Read the model definition and answer for the solid it produces. Units are mm, in the model's axes. A direction names the side the tool comes from. Give positions to 0.01 mm unless a question says otherwise; leave off trailing zeros. Write each loop counter-clockwise with the first axis right and the second up, starting at its lowest first coordinate (ties: lowest second). Pieces come first, ordered by that corner, then holes. Notation, with made-up numbers: M -5,53.5 L 22,53.5 A18 ccw 22,75.5 Z; hole C 78.25,39 d7. An arc over 180 degrees is marked long. Answer as CSV lines item,"result". Start each with the question number.
```python
from build123d import *

# Parameters (mm, degrees)
BOSS_EXTRUDE1_DEPTH = 8
SKETCH3_W           = 84
SKETCH3_H           = 8
BOSS_EXTRUDE3_DEPTH = 3
SKETCH4_R           = 1.8
CUT_EXTRUDE1_DEPTH  = 44.9089968
SKETCH5_R           = 1.8
CUT_EXTRUDE2_DEPTH  = 44.9089968
SKETCH6_R           = 3.75
CUT_EXTRUDE3_DEPTH  = 6


with BuildPart() as part:
    # Sketch2 → Boss-Extrude1 (new body)
    with BuildSketch(Plane(origin=(0, 0, 0), x_dir=(1, 0, 0), z_dir=(0, 1, 0))):
        Polygon((-10, 0), (10, 0), (20, -10), (-20, -10), align=None)
    extrude(amount=BOSS_EXTRUDE1_DEPTH)

    # Sketch3 → Boss-Extrude3 (add)
    with BuildSketch(Plane.XY.offset(10)):
        with Locations((0, 4)):
            Rectangle(SKETCH3_W, SKETCH3_H)
    extrude(amount=-BOSS_EXTRUDE3_DEPTH)

    # Sketch4 → Cut-Extrude1 (cut, through all)
    with BuildSketch(Plane.XY.offset(10)):
        with Locations((-38.15, 4)):
            Circle(SKETCH4_R)
        with Locations((38.15, 4)):
            Circle(SKETCH4_R)
    extrude(amount=-CUT_EXTRUDE1_DEPTH, mode=Mode.SUBTRACT)

    # Sketch5 → Cut-Extrude2 (cut, through all)
    with BuildSketch(Plane(origin=(0, 0, 0), x_dir=(-1, 0, 0), z_dir=(0, 0, -1))):
        with Locations((0, 4)):
            Circle(SKETCH5_R)
    extrude(amount=-CUT_EXTRUDE2_DEPTH, mode=Mode.SUBTRACT)

    # Sketch6 → Cut-Extrude3 (cut)
    with BuildSketch(Plane.XY.offset(10)):
        with Locations((0, 4)):
            Circle(SKETCH6_R)
    extrude(amount=-CUT_EXTRUDE3_DEPTH, mode=Mode.SUBTRACT)


solid = part.part
```
1. Given pin 1 (2 mm diameter, centred on x = 0, y = 4, fed in from -Z); pin 2 (1.5 mm diameter, centred on y = 7, z = 5.5, fed in from +X); pin 3 (2 mm diameter, centred on x = 2, y = 2.5, fed in from +Z); pin 4 (4 mm diameter, centred on x = 38.15, y = 4, fed in from -Z), each flat-ended and moving along its own axis, determine where each tip first touches the part or whether it passes through.
2. Find section D-D on z = 1.5. Determine the outline of the cut face in (x, y), then the cut area to 3 significant figures.
3. For faces 4 (the face through (-30, 4, 7)), 5 (the face through (29, 4, 7)), 6 (the face through (-0.81, 0.34, 7.04)), determine the directions among +Z, -Z, +X, -X, +Y, -Y from which every point of the face is accessible in a straight line to the end or side of a thin tool.
4. Determine the mould class of faces 1 (the face through (9, 4, 10)), 2 (the face through (13, 4, 3)), 3 (the face through (-1, 2, 4)) for opening direction X: +X half, -X half, draft (parallel to the pull), parting line (faces both ways), or undercut.
5. Find section A-A on x = -38.15. Determine the outline of the cut face in (y, z).
6. Find section B-B on z = 8.5. Determine the outline of the cut face in (x, y), then the cut area to 3 significant figures.
7. Find the intervals of material crossed by line 1 (Y direction, x = 38.15, z = 8.6); line 2 (Y direction, x = 0, z = 8.7); line 3 (Z direction, x = -29, y = 4), in increasing order. Write a range as [from, to].
8. Find section C-C on y = 4. Determine the outline of the cut face in (x, z).
Computed:
1,pin 1,"passes through"
1,pin 2,"stops at x = 16.25"
1,pin 3,"stops at z = 4"
1,pin 4,"stops at z = 7"
2,outline,"M -11.5,0 L 11.5,0 L 11.5,8 L -11.5,8 Z; hole C 0,4 d3.6"
2,area,"174 mm^2"
3,face 4,"-Z, -X, +Y, -Y"
3,face 5,"-Z, +X, +Y, -Y"
3,face 6,"+Z"
4,face 1,"draft"
4,face 2,"+X half"
4,face 3,"undercut"
5,outline,"M 0,7 L 2.2,7 L 2.2,10 L 0,10 Z; M 5.8,7 L 8,7 L 8,10 L 5.8,10 Z"
6,outline,"M -42,0 L 42,0 L 42,8 L -42,8 Z; hole C -38.15,4 d3.6; hole C 0,4 d7.5; hole C 38.15,4 d3.6"
6,area,"607 mm^2"
7,line 1,"y = [0, 2.2], [5.8, 8]"
7,line 2,"y = [0, 0.25], [7.75, 8]"
7,line 3,"z = [7, 10]"
8,outline,"M -42,7 L -39.95,7 L -39.95,10 L -42,10 Z; M -36.35,7 L -17,7 L -10,0 L -1.8,0 L -1.8,4 L -3.75,4 L -3.75,10 L -36.35,10 Z; M 1.8,0 L 10,0 L 17,7 L 36.35,7 L 36.35,10 L 3.75,10 L 3.75,4 L 1.8,4 Z; M 39.95,7 L 42,7 L 42,10 L 39.95,10 Z"
